```python
from build123d import *

# Parameters (mm, degrees)
SKETCH1_R           = 25.000000000000004
SKETCH1_R_2         = 1.9999999999993712
SKETCH1_R_3         = 2.0000000000000036
SKETCH1_R_4         = 2.0000000000002736
SKETCH1_R_5         = 1.9999999999996778
BOSS_EXTRUDE1_DEPTH = 4
SKETCH2_R           = 25
SKETCH2_R_2         = 22.50000000000001
BOSS_EXTRUDE2_DEPTH = 15
BOSS_EXTRUDE7_REACH = 78.843
SKETCH4_W           = 49.955357531530346
SKETCH4_H           = 19
BOSS_EXTRUDE8_DEPTH = 4
SKETCH7_R           = 2.499999999999995
SKETCH7_R_2         = 2.5000000000000004
CUT_EXTRUDE1_DEPTH  = 4
FILLET1_R           = 5
FILLET2_R           = 5


with BuildPart() as part:
    # Sketch1 → Boss-Extrude1 (new body)
    with BuildSketch(Plane(origin=(0, 0, 0), x_dir=(1, 0, 0), z_dir=(0, 1, 0))):
        with Locations(Location((21.22072875619714, -40.09390888269783, 0), (0, 0, 270))):
            Circle(SKETCH1_R)
        with Locations(Location((29.646509797315062, -55.43197309716617, 0), (0, 0, 270))):
            Circle(SKETCH1_R_2, mode=Mode.SUBTRACT)
        with Locations(Location((36.558792970665294, -31.668127841580553, 0), (0, 0, 270))):
            Circle(SKETCH1_R_3, mode=Mode.SUBTRACT)
        with Locations(Location((12.794947715079665, -24.75584466823032, 0), (0, 0, 270))):
            Circle(SKETCH1_R_4, mode=Mode.SUBTRACT)
        with Locations(Location((5.8826645417294365, -48.51968992381595, 0), (0, 0, 270))):
            Circle(SKETCH1_R_5, mode=Mode.SUBTRACT)
        with BuildLine():
            ThreePointArc((8.810101512256844, -41.5859984952772), (17.729498538084204, -52.096463259335145), (30.894801565269475, -48.009862096604984))
            Line((30.894801565269475, -48.009862096604984), (33.63135600013741, -38.60181927011846))
            ThreePointArc((33.63135600013741, -38.60181927011846), (24.711958974310075, -28.091354506060547), (11.5466559471248, -32.177955668790645))
            Line((11.5466559471248, -32.177955668790645), (8.810101512256844, -41.5859984952772))
        make_face(mode=Mode.SUBTRACT)
    extrude(amount=BOSS_EXTRUDE1_DEPTH)

    # Sketch2 → Boss-Extrude2 (add)
    with BuildSketch(Plane.XZ):
        with Locations(Location((21.22070938805554, 40.093908619998004, 0), (0, 0, 270.77710591))):
            Circle(SKETCH2_R)
        with Locations(Location((21.22070938805554, 40.093908619998004, 0), (0, 0, 270))):
            Circle(SKETCH2_R_2, mode=Mode.SUBTRACT)
    extrude(amount=BOSS_EXTRUDE2_DEPTH)

    # Sketch4 → Boss-Extrude7 (add, up to next)
    with BuildSketch(Plane(origin=(-2.11468835096776, 0, 7.270119796296657), x_dir=(-0.9602043501309836, 0, -0.2792984174490354), z_dir=(0.2792984174490354, 0, -0.9602043501309836)), mode=Mode.PRIVATE) as boss_extrude7_sk1:
        with Locations((-31.573501878114026, -5.500000000000001)):
            Rectangle(SKETCH4_W, SKETCH4_H)
    boss_extrude7_tool1 = extrude(boss_extrude7_sk1.sketch, amount=-BOSS_EXTRUDE7_REACH, mode=Mode.PRIVATE) - part.part
    add(boss_extrude7_tool1.solids().sort_by_distance((28.202326, -5.5, 16.088549))[0])

    # Sketch5 → Boss-Extrude8 (add)
    with BuildSketch(Plane(origin=(-2.114688350967763, 0, 7.270119796296668), x_dir=(-0.9602043501309836, 0, -0.27929841744903544), z_dir=(0.27929841744903544, 0, -0.9602043501309836))):
        Polygon((13.404176887651147, 4), (-76.55118064387919, 4), (-76.55118064387919, -15), (13.404176887651147, -15), (13.404176887651147, -5.5), align=None)
    extrude(amount=BOSS_EXTRUDE8_DEPTH)

    # Sketch7 → Cut-Extrude1 (cut)
    with BuildSketch(Plane(origin=(-0.9974946811716227, -2e-16, 3.4293023957727353), x_dir=(-0.9602043501309836, 0, -0.27929841744903544), z_dir=(0.27929841744903544, 0, -0.9602043501309836))):
        with Locations((-66.55118064387919, -5.499999999999998)):
            Circle(SKETCH7_R)
        with Locations((3.4041768876511456, -5.499999999999997)):
            Circle(SKETCH7_R_2)
    extrude(amount=-CUT_EXTRUDE1_DEPTH, mode=Mode.SUBTRACT)

    # Fillet1
    fillet1_edges = [part.edges().sort_by_distance(p)[0] for p in [
        (71.94868514584586, -15, 26.730334703725394),
    ]]
    fillet(fillet1_edges, radius=FILLET1_R)

    # Fillet2
    fillet2_edges = [part.edges().sort_by_distance(p)[0] for p in [
        (-14.426840473517512, -15, 1.605945704106798),
        (-14.426840473517512, 4, 1.605945704106798),
        (71.94868514584586, 4, 26.730334703725394),
    ]]
    fillet(fillet2_edges, radius=FILLET2_R)


solid = part.part
```
Work out the finished part from the listing and answer in its coordinate system (mm). A direction names the side the tool comes from. Give positions to 0.01 mm unless a question says otherwise; leave off trailing zeros. Loops run counter-clockwise (first coordinate to the right, second up) from the corner with the lowest first, then second, coordinate; pieces in that order, holes last. Notation, with made-up numbers: (-39, 85) -> (1, 85) arc R21 cw to (1, 94) -> close; hole circle Ø2 at (18, 54.25). An arc over 180 degrees is marked (long way). One line per question, with ' | ' between items. Start each with the question number.
1) Determine the mould class of faces 1 (the face through (-12.98, -13.57, 2)), 2 (the face through (70.587, 2.496, 26.305)), 3 (the face through (-3.115, -3.256, 6.979)) for opening direction Z: +Z half, -Z half, draft (parallel to the pull), parting line (faces both ways), or undercut.
2) Each of these flat-tipped pins is pushed along its axis until it touches: pin 1 (5.5 mm diameter, centred on x = 28.5, z = 57.5, fed in from -Y); pin 2 (3 mm diameter, centred on y = -8, z = 24, fed in from -X); pin 3 (10 mm diameter, centred on y = -9.5, z = 29, fed in from -X); pin 4 (3 mm diameter, centred on x = 36.56, z = 31.67, fed in from +Y). Where does it stop, or does it pass through?
3) Straight lines are drawn through the part: L1, parallel to X at y = -3.25, z = 36.5; L2, parallel to Z at x = 6, y = 3; L3, parallel to Z at x = 29, y = -2.25. For each, find the intervals that lie inside material, in ascending order.
4) Section A-A, the plane y = -4.25 is taken. Determine the outline of the cut face in (x, z), then the cut area to 3 significant figures.
5) Section D-D, the plane z = 31 is taken. Determine the outline of the cut face in (x, y), then the cut area to 3 significant figures.
6) For faces 4 (the face through (48.89, -5.63, 34.39)), 5 (the face through (24.91, 1.97, 28.15)), 6 (the face through (12, 0, 50)), determine the directions among +Z, -Z, +X, -X, +Y, -Y from which every point of the face is accessible in a straight line to the end or side of a thin tool.
Resolved:
1) face 1: -Z half | face 2: +Z half | face 3: undercut
2) pin 1: y = 0 | pin 2: x = -0.55 | pin 3: x = -3.03 | pin 4: through
3) L1: -3.52 to -0.99, 43.43 to 48.28 | L2: 5.46 to 46.52, 50.52 to 59.93 | L3: 12.15 to 18.98, 61.21 to 63.85
4) outline: (-14.99, 3.53) -> (-13.87, -0.31) -> (-6.35, 1.87) -> (-7.46, 5.71) -> close; (-3.3, 6.92) -> (-2.19, 3.08) -> (60.83, 21.41) -> (59.71, 25.25) -> (52.19, 23.06) -> (45.5, 46.04) arc R25 ccw (long way) to (-2.47, 32.12) -> (4.22, 9.11) -> close; (63.87, 26.46) -> (64.98, 22.62) -> (72.51, 24.81) -> (71.39, 28.65) -> close; hole circle Ø45 at (21.22, 40.09) | area: 965 mm2
5) outline: (-2.15, -15) -> (0.64, -15) -> (0.64, 0) -> (12.64, 0) -> (12.64, 4) -> (-2.15, 4) -> close; (29.8, 0) -> (34.67, 0) -> (34.67, 4) -> (29.8, 4) -> close; (38.44, 0) -> (41.8, 0) -> (41.8, -15) -> (49.88, -15) -> (49.88, 4) -> (38.44, 4) -> close | area: 287 mm2
6) face 4: +Z, +Y, -Y | face 5: +Y, -Y | face 6: -Y
